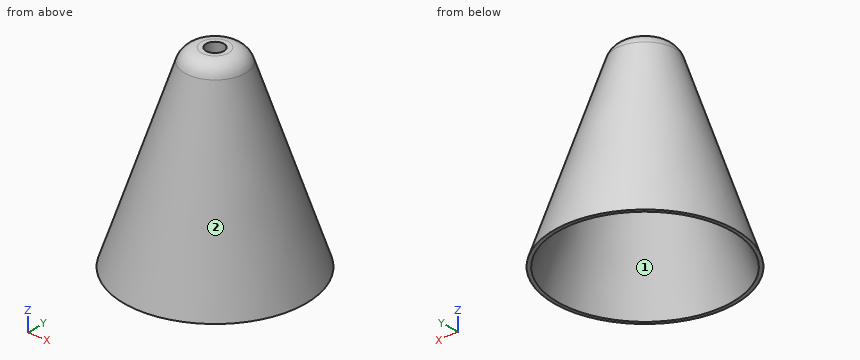
```python
from build123d import *

# Parameters (mm, degrees)
F0_R      = 52
F4_R      = 15
F2_R      = 20
F6_R      = 50
F9_R      = 5.125
F10_DEPTH = 25
F11_R     = 10
F12_R     = 9.4


with BuildPart() as f5:
    # F0 (on Top) → F5 section 0
    with BuildSketch(Plane.XY):
        Circle(F0_R)
    # F4 (on offset) → F5 section 1
    with BuildSketch(Plane.XY.offset(110)):
        Circle(F4_R)
    loft()

    # F2 (on offset) → F7 section 0
    with BuildSketch(Plane.XY.offset(80)):
        Circle(F2_R)
    # F6 (on face) → F7 section 1
    with BuildSketch(Plane(origin=(0, 0, 0), x_dir=(1, 0, 0), z_dir=(0, 0, -1))):
        Circle(F6_R)
    loft(mode=Mode.SUBTRACT)

    # F9 (on face) → F10 (cut)
    with BuildSketch(Plane.XY.offset(110)):
        Circle(F9_R)
    extrude(amount=-F10_DEPTH, mode=Mode.SUBTRACT)

    # F11
    f11_edges = [f5.edges().sort_by_distance(p)[0] for p in [
        (-15, 0, 110),
    ]]
    fillet(f11_edges, radius=F11_R)

    # F12
    f12_edges = [f5.edges().sort_by_distance(p)[0] for p in [
        (-20, 0, 80),
    ]]
    fillet(f12_edges, radius=F12_R)


solid = f5.part
```
CAD build for the part. Positions are in the model's coordinates, mm. Face numbers are marked on the shaded views. Give positions to 0.01 mm unless a question says otherwise; leave off trailing zeros. Order: outer loops, then holes, each group sorted by start corner. A loop starts at its lowest first (then second) coordinate and runs counter-clockwise, first axis right, second up.
(1) Mould opens along Y. For the marked faces 1 and 2 say: released by +Y, released by -Y, zero draft, split by the parting line, or undercut.
(2) Saw through at A-A, the plane z = 45. Give the cut face in (x, y) (3 decimals), then the cut area to 3 significant figures.
(3) Flat gauge pins, fed straight in: pin 1 (4 mm diameter, centred on y = 20, z = 19, fed in from +X); pin 2 (8 mm diameter, centred on x = 1, y = 6.5, fed in from -Z); pin 3 (5 mm diameter, centred on x = -1, y = 0, fed in from +Z). Where does each tip first touch, or does it go through?
(4) Drill centre lines: L1, parallel to Y at x = 0, z = 93.5 (3 decimals); L2, parallel to Y at x = -7, z = 70; L3, parallel to X at y = -25, z = 55. Where is each one in solid material? Low to high.
(5) Saw through at B-B, the plane z = 87. Give the cut face in (x, y) (3 decimals), then the cut area to 3 significant figures.
Results found:
1. face 1: undercut
1. face 2: split by the parting line
2. outline: circle Ø73.727 at (0, 0); hole circle Ø66.25 at (0, 0)
2. area: 822 mm2
3. pin 1: stops at x = 42.18
3. pin 2: stops at z = 80
3. pin 3: stops at z = 85
4. L1: y = -20.55 to -5.125, 5.125 to 20.55
4. L2: y = -27.58 to -22.69, 22.69 to 27.58
4. L3: x = -22.3 to -15.42, 15.42 to 22.3
5. outline: circle Ø45.473 at (0, 0); hole circle Ø10.25 at (0, 0)
5. area: 1,540 mm2
